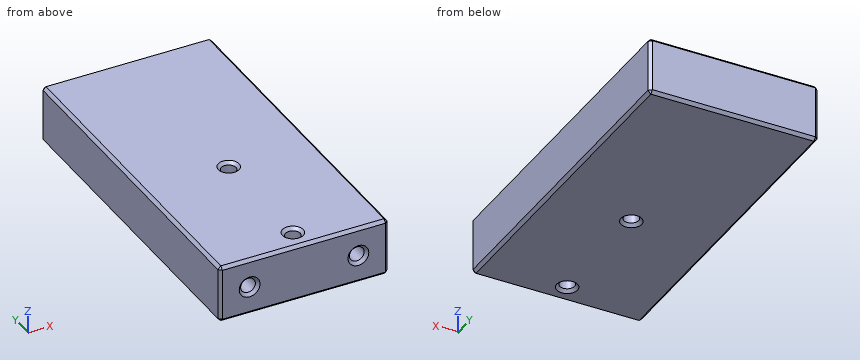
```python
from build123d import *

# Parameters (mm, degrees)
SKETCH1_W           = 28
SKETCH1_H           = 55.475
BOSS_EXTRUDE1_DEPTH = 9.525
SKETCH2_R           = 1.2195
CUT_EXTRUDE1_DEPTH  = 20
SKETCH3_R           = 1.2195
CUT_EXTRUDE2_DEPTH  = 63.866535215
CHAMFER1_SIZE       = 0.5
CHAMFER2_SIZE       = 0.5


with BuildPart() as part:
    # Sketch1 → Boss-Extrude1 (new body)
    with BuildSketch(Plane.XY):
        with Locations((14, 27.7375)):
            Rectangle(SKETCH1_W, SKETCH1_H)
    extrude(amount=BOSS_EXTRUDE1_DEPTH)

    # Sketch2 → Cut-Extrude1 (cut)
    with BuildSketch(Plane.XZ):
        with Locations(Location((5, 4.7625, 0), (0, 0, 270))):
            Circle(SKETCH2_R)
        with Locations(Location((23, 4.7625, 0), (0, 0, 270))):
            Circle(SKETCH2_R)
    extrude(amount=-CUT_EXTRUDE1_DEPTH, mode=Mode.SUBTRACT)

    # Sketch3 → Cut-Extrude2 (cut, through all)
    with BuildSketch(Plane.XY.offset(9.525)):
        with Locations((14, 23.475)):
            Circle(SKETCH3_R)
        with Locations((14, 3.475)):
            Circle(SKETCH3_R)
    extrude(amount=-CUT_EXTRUDE2_DEPTH, mode=Mode.SUBTRACT)

    # Chamfer1
    chamfer1_edges = [part.edges().sort_by_distance(p)[0] for p in [
        (28, 27.7375, 9.525),
        (14, 55.475, 9.525),
        (0, 27.7375, 9.525),
        (14, 55.475, 0),
        (28, 27.7375, 0),
        (14, 0, 0),
        (0, 27.7375, 0),
        (14, 0, 9.525),
        (0, 55.475, 4.7625),
        (28, 55.475, 4.7625),
        (28, 0, 4.7625),
        (0, 0, 4.7625),
    ]]
    chamfer(chamfer1_edges, length=CHAMFER1_SIZE)

    # Chamfer2
    chamfer2_edges = [part.edges().sort_by_distance(p)[0] for p in [
        (5, 0, 5.982),
        (23, 0, 5.982),
        (12.7805, 23.475, 0),
        (12.7805, 23.475, 9.525),
        (12.7805, 3.475, 0),
        (12.7805, 3.475, 9.525),
    ]]
    chamfer(chamfer2_edges, length=CHAMFER2_SIZE)


solid = part.part
```
Input: part model. Units: mm. Frame: model coordinates. Coordinates: 2 decimals unless noted, no trailing zeros. Order: outer loops, then holes, each group sorted by start corner. A loop starts at its lowest first (then second) coordinate and runs counter-clockwise, first axis right, second up. Notation, with made-up numbers: (4, 7) - (13, 7) arc R24 cw to (13, 37) - close; hole circle Ø2 at (71.25, 73). An arc over 180 degrees is marked (long way). Put each result on its own line as item: value.
1. Cut plane B-B on y = 10.5. Return the cut outline in (x, z) (1 decimal).
Report:
outline: (0, 0.5) - (0.5, 0) - (27.5, 0) - (28, 0.5) - (28, 9) - (27.5, 9.5) - (0.5, 9.5) - (0, 9) - close; hole circle Ø2.4 at (5, 4.8); hole circle Ø2.4 at (23, 4.8)
2. Line query: line 1 along Y through (x, z) = (14, 2.25) (1 decimal); line 2 along X through (y, z) = (4, 5.75); line 3 along X through (y, z) = (3, 1.75). Output: solid intervals per line, ascending.
Report:
line 1: y = 0 to 2.3, 4.7 to 22.3, 24.7 to 55.5
line 2: x = 0 to 4.28, 5.72 to 12.9, 15.1 to 22.28, 23.72 to 28
line 3: x = 0 to 12.88, 15.12 to 28
3. Cut plane C-C on x = 5. Return the cut outline in (y, z) (3 decimals), then the cut area to 3 significant figures.
Report:
outline: (0, 0.5) - (0.5, 0) - (54.975, 0) - (55.475, 0.5) - (55.475, 9.025) - (54.975, 9.525) - (0.5, 9.525) - (0, 9.025) - (0, 6.482) - (0.5, 5.982) - (20, 5.982) - (20, 3.543) - (0.5, 3.543) - (0, 3.043) - close
area: 479 mm2
4. Contact query for flat-ended pins moving along their axis: pin 1 Ø3 at (x, y) = (14, 3.475) entering from -Z; pin 2 Ø3 at (x, y) = (14, 23.475) entering from +Z; pin 3 Ø0.7 at (x, z) = (4.5, 4.5) entering from -Y. Output: stop coordinate, or through.
Report:
pin 1: stops at z = 0.22
pin 2: stops at z = 9.31
pin 3: stops at y = 20
5. Cut plane A-A on x = 14. Return the cut outline in (y, z) (1 decimal), then the cut area to 3 significant figures.
Report:
outline: (0, 0.5) - (0.5, 0) - (1.8, 0) - (2.3, 0.5) - (2.3, 9) - (1.8, 9.5) - (0.5, 9.5) - (0, 9) - close; (4.7, 0.5) - (5.2, 0) - (21.8, 0) - (22.3, 0.5) - (22.3, 9) - (21.8, 9.5) - (5.2, 9.5) - (4.7, 9) - close; (24.7, 0.5) - (25.2, 0) - (55, 0) - (55.5, 0.5) - (55.5, 9) - (55, 9.5) - (25.2, 9.5) - (24.7, 9) - close
area: 480 mm2
